```python
from build123d import *

# Parameters (mm, degrees)
SALIENTE_EXTRUIR1_DEPTH = 4
CROQUIS3_W              = 28.5
CROQUIS3_H              = 75
CORTAR_EXTRUIR1_DEPTH   = 135.40982107
CROQUIS4_R              = 2.25
CROQUIS4_R_2            = 2.1
CORTAR_EXTRUIR2_DEPTH   = 135.40982107
CROQUIS5_R              = 25
CORTAR_EXTRUIR3_DEPTH   = 135.40982107
REDONDEO1_R             = 5
CROQUIS6_R              = 2.1
CORTAR_EXTRUIR4_DEPTH   = 135.40982107
CROQUIS7_R              = 2.1
CORTAR_EXTRUIR5_DEPTH   = 135.40982107
CORTAR_EXTRUIR6_REACH   = 136.41
CROQUIS8_R              = 2.1
CROQUIS9_R              = 2.1
CORTAR_EXTRUIR7_DEPTH   = 135.40982107


with BuildPart() as part:
    # Croquis2 → Saliente-Extruir1 (new body)
    with BuildSketch(Plane(origin=(0, 0, 0), x_dir=(1, 0, 0), z_dir=(0, 1, 0))):
        Polygon((-65, 95), (-95, 80), (-95, -95), (95, -95), (95, 80), (65, 95), align=None)
    extrude(amount=SALIENTE_EXTRUIR1_DEPTH)

    # Croquis3 → Cortar-Extruir1 (cut, through all)
    with BuildSketch(Plane(origin=(0, 4, 0), x_dir=(1, 0, 0), z_dir=(0, 1, 0))):
        with Locations((-80.75, 35)):
            Rectangle(CROQUIS3_W, CROQUIS3_H)
        with Locations((80.75, 35)):
            Rectangle(CROQUIS3_W, CROQUIS3_H)
    extrude(amount=-CORTAR_EXTRUIR1_DEPTH, mode=Mode.SUBTRACT)

    # Croquis4 → Cortar-Extruir2 (cut, through all)
    with BuildSketch(Plane(origin=(0, 4, 0), x_dir=(1, 0, 0), z_dir=(0, 1, 0))):
        with Locations(Location((-80.75, -19.5, 0), (0, 0, 270))):
            Circle(CROQUIS4_R)
        with Locations(Location((-80.75, -34.5, 0), (0, 0, 270))):
            Circle(CROQUIS4_R)
        with Locations(Location((-80.75, -49.5, 0), (0, 0, 270))):
            Circle(CROQUIS4_R)
        with Locations(Location((-56.5, 80.75, 0), (0, 0, 270))):
            Circle(CROQUIS4_R_2)
        with Locations(Location((-41.5, 80.75, 0), (0, 0, 270))):
            Circle(CROQUIS4_R_2)
        with Locations(Location((-26.5, 80.75, 0), (0, 0, 270))):
            Circle(CROQUIS4_R_2)
        with Locations(Location((80.75, -49.5, 0), (0, 0, 90))):
            Circle(CROQUIS4_R)
        with Locations(Location((80.75, -34.5, 0), (0, 0, 90))):
            Circle(CROQUIS4_R)
        with Locations(Location((80.75, -19.5, 0), (0, 0, 90))):
            Circle(CROQUIS4_R)
        with Locations(Location((26.5, 80.75, 0), (0, 0, 90))):
            Circle(CROQUIS4_R_2)
        with Locations(Location((41.5, 80.75, 0), (0, 0, 90))):
            Circle(CROQUIS4_R_2)
        with Locations(Location((56.5, 80.75, 0), (0, 0, 90))):
            Circle(CROQUIS4_R_2)
    extrude(amount=-CORTAR_EXTRUIR2_DEPTH, mode=Mode.SUBTRACT)

    # Croquis5 → Cortar-Extruir3 (cut, through all)
    with BuildSketch(Plane(origin=(0, 4, 0), x_dir=(1, 0, 0), z_dir=(0, 1, 0))):
        with Locations(Location((0, 35, 0), (0, 0, 270))):
            Circle(CROQUIS5_R)
        with BuildLine():
            Line((-20, -21.536154127), (-20, -66.536154127))
            ThreePointArc((-20, -66.536154127), (-30, -76.536154127), (-40, -66.536154127))
            Line((-40, -66.536154127), (-40, -21.536154127))
            ThreePointArc((-40, -21.536154127), (-30, -11.536154127), (-20, -21.536154127))
        make_face()
        with BuildLine():
            Line((20, -21.536154127), (20, -66.536154127))
            ThreePointArc((20, -66.536154127), (30, -76.536154127), (40, -66.536154127))
            Line((40, -66.536154127), (40, -21.536154127))
            ThreePointArc((40, -21.536154127), (30, -11.536154127), (20, -21.536154127))
        make_face()
    extrude(amount=-CORTAR_EXTRUIR3_DEPTH, mode=Mode.SUBTRACT)

    # Redondeo1
    # the kernel refuses this fillet: 5 mm, written as the material it adds along each edge
    with BuildSketch(Plane(origin=(-66.5, 4, -72.5), x_dir=(-1, 0, 0), z_dir=(0, -1, 0)), Plane(origin=(-66.5, 4, 2.5), x_dir=(0, 0, -1), z_dir=(0, -1, 0))) as redondeo1_piece_1:
        with BuildLine():
            CenterArc((REDONDEO1_R, -REDONDEO1_R), REDONDEO1_R, 90, 90)
            Line((0, -REDONDEO1_R), (0, 0))
            Line((0, 0), (REDONDEO1_R, 0))
        make_face()
    extrude(amount=4)
    with BuildSketch(Plane(origin=(66.5, 4, -72.5), x_dir=(1, 0, 0), z_dir=(0, -1, 0)), Plane(origin=(66.5, 4, 2.5), x_dir=(0, 0, -1), z_dir=(0, -1, 0))) as redondeo1_piece_2:
        with BuildLine():
            CenterArc((REDONDEO1_R, REDONDEO1_R), REDONDEO1_R, 180, 90)
            Line((0, REDONDEO1_R), (0, 0))
            Line((0, 0), (REDONDEO1_R, 0))
        make_face()
    extrude(amount=4)
    # the kernel refuses this fillet: 5 mm, written as the material it takes off along each edge
    with BuildSketch(Plane(origin=(95, -12.5, 95), x_dir=(0, 0, -1), z_dir=(0, 1, 0)), Plane(origin=(-95, -12.5, 95), x_dir=(1, 0, 0), z_dir=(0, 1, 0)), Plane(origin=(-95, 16.5, -72.5), x_dir=(0, 0, -1), z_dir=(0, -1, 0))) as redondeo1_2_piece_1:
        with BuildLine():
            CenterArc((REDONDEO1_R, REDONDEO1_R), REDONDEO1_R, 180, 90)
            Line((0, REDONDEO1_R), (0, 0))
            Line((0, 0), (REDONDEO1_R, 0))
        make_face()
    extrude(amount=29, mode=Mode.SUBTRACT)
    with BuildSketch(Plane(origin=(-95, -7.725424859, -80), x_dir=(0.894427190999916, 0, -0.447213595499958), z_dir=(0, 1, 0))) as redondeo1_2_piece_2:
        with BuildLine():
            CenterArc((REDONDEO1_R * 0.61803398875, -REDONDEO1_R), REDONDEO1_R, 90, 63.434948823)
            Line((-REDONDEO1_R * 0.27639320225, -REDONDEO1_R * 0.5527864045), (0, 0))
            Line((0, 0), (REDONDEO1_R * 0.61803398875, 0))
        make_face()
    extrude(amount=19.450849719, mode=Mode.SUBTRACT)
    with BuildSketch(Plane(origin=(-65, -2.950849719, -95), x_dir=(1, 0, 0), z_dir=(0, 1, 0)), Plane(origin=(65, -2.950849719, -95), x_dir=(0.8944271909999183, 0, 0.44721359549995315), z_dir=(0, 1, 0))) as redondeo1_2_piece_3:
        with BuildLine():
            CenterArc((REDONDEO1_R * 0.2360679775, -REDONDEO1_R), REDONDEO1_R, 90, 26.565051177)
            Line((-REDONDEO1_R * 0.211145618, -REDONDEO1_R * 0.105572809), (0, 0))
            Line((0, 0), (REDONDEO1_R * 0.2360679775, 0))
        make_face()
    extrude(amount=9.901699437, mode=Mode.SUBTRACT)
    with BuildSketch(Plane(origin=(95, -7.725424859, -80), x_dir=(-0.894427190999915, 0, -0.4472135954999598), z_dir=(0, 1, 0))) as redondeo1_2_piece_4:
        with BuildLine():
            CenterArc((REDONDEO1_R * 0.61803398875, REDONDEO1_R), REDONDEO1_R, 206.565051177, 63.434948823)
            Line((-REDONDEO1_R * 0.27639320225, REDONDEO1_R * 0.5527864045), (0, 0))
            Line((0, 0), (REDONDEO1_R * 0.61803398875, 0))
        make_face()
    extrude(amount=19.450849719, mode=Mode.SUBTRACT)
    with BuildSketch(Plane(origin=(-95, 16.5, 2.5), x_dir=(0, 0, 1), z_dir=(0, -1, 0)), Plane(origin=(95, 16.5, -72.5), x_dir=(0, 0, -1), z_dir=(0, -1, 0)), Plane(origin=(95, 16.5, 2.5), x_dir=(-1, 0, 0), z_dir=(0, -1, 0))) as redondeo1_2_piece_5:
        with BuildLine():
            CenterArc((REDONDEO1_R, -REDONDEO1_R), REDONDEO1_R, 90, 90)
            Line((0, -REDONDEO1_R), (0, 0))
            Line((0, 0), (REDONDEO1_R, 0))
        make_face()
    extrude(amount=29, mode=Mode.SUBTRACT)

    # Croquis6 → Cortar-Extruir4 (cut, through all)
    with BuildSketch(Plane(origin=(0, 4, 0), x_dir=(1, 0, 0), z_dir=(0, 1, 0))):
        with Locations(Location((-57.5, -85, 0), (0, 0, 270))):
            Circle(CROQUIS6_R)
        with Locations(Location((-42.5, -85, 0), (0, 0, 270))):
            Circle(CROQUIS6_R)
        with Locations(Location((42.5, -85, 0), (0, 0, 90))):
            Circle(CROQUIS6_R)
        with Locations(Location((57.5, -85, 0), (0, 0, 90))):
            Circle(CROQUIS6_R)
        with Locations(Location((-7.5, -85, 0), (0, 0, 270))):
            Circle(CROQUIS6_R)
        with Locations(Location((7.5, -85, 0), (0, 0, 270))):
            Circle(CROQUIS6_R)
    extrude(amount=-CORTAR_EXTRUIR4_DEPTH, mode=Mode.SUBTRACT)

    # Croquis7 → Cortar-Extruir5 (cut, through all)
    with BuildSketch(Plane(origin=(0, 4, 0), x_dir=(1, 0, 0), z_dir=(0, 1, 0))):
        with Locations(Location((-57.5, -70, 0), (0, 0, 270))):
            Circle(CROQUIS7_R)
        with Locations(Location((-57.5, -55, 0), (0, 0, 270))):
            Circle(CROQUIS7_R)
        with Locations(Location((57.5, -55, 0), (0, 0, 90))):
            Circle(CROQUIS7_R)
        with Locations(Location((57.5, -70, 0), (0, 0, 90))):
            Circle(CROQUIS7_R)
        with Locations(Location((0, -70, 0), (0, 0, 270))):
            Circle(CROQUIS7_R)
        with Locations(Location((0, -55, 0), (0, 0, 270))):
            Circle(CROQUIS7_R)
    extrude(amount=-CORTAR_EXTRUIR5_DEPTH, mode=Mode.SUBTRACT)

    # Croquis8 → Cortar-Extruir6 (cut, up to next)
    with BuildSketch(Plane.XZ, mode=Mode.PRIVATE) as cortar_extruir6_sk1:
        with Locations(Location((56.5, -57.25, 0), (0, 0, 270))):
            Circle(CROQUIS8_R)
    cortar_extruir6_tool1 = extrude(cortar_extruir6_sk1.sketch, amount=-CORTAR_EXTRUIR6_REACH, mode=Mode.PRIVATE) & part.part
    # Croquis8 → Cortar-Extruir6 (cut, up to next)
    with BuildSketch(Plane.XZ, mode=Mode.PRIVATE) as cortar_extruir6_sk2:
        with Locations(Location((36.5, -57.25, 0), (0, 0, 270))):
            Circle(CROQUIS8_R)
    cortar_extruir6_tool2 = extrude(cortar_extruir6_sk2.sketch, amount=-CORTAR_EXTRUIR6_REACH, mode=Mode.PRIVATE) & part.part
    # Croquis8 → Cortar-Extruir6 (cut, up to next)
    with BuildSketch(Plane.XZ, mode=Mode.PRIVATE) as cortar_extruir6_sk3:
        with Locations(Location((56.5, -12.75, 0), (0, 0, 90))):
            Circle(CROQUIS8_R)
    cortar_extruir6_tool3 = extrude(cortar_extruir6_sk3.sketch, amount=-CORTAR_EXTRUIR6_REACH, mode=Mode.PRIVATE) & part.part
    # Croquis8 → Cortar-Extruir6 (cut, up to next)
    with BuildSketch(Plane.XZ, mode=Mode.PRIVATE) as cortar_extruir6_sk4:
        with Locations(Location((36.5, -12.75, 0), (0, 0, 90))):
            Circle(CROQUIS8_R)
    cortar_extruir6_tool4 = extrude(cortar_extruir6_sk4.sketch, amount=-CORTAR_EXTRUIR6_REACH, mode=Mode.PRIVATE) & part.part
    # Croquis8 → Cortar-Extruir6 (cut, up to next)
    with BuildSketch(Plane.XZ, mode=Mode.PRIVATE) as cortar_extruir6_sk5:
        with Locations(Location((-36.5, -12.75, 0), (0, 0, 270))):
            Circle(CROQUIS8_R)
    cortar_extruir6_tool5 = extrude(cortar_extruir6_sk5.sketch, amount=-CORTAR_EXTRUIR6_REACH, mode=Mode.PRIVATE) & part.part
    # Croquis8 → Cortar-Extruir6 (cut, up to next)
    with BuildSketch(Plane.XZ, mode=Mode.PRIVATE) as cortar_extruir6_sk6:
        with Locations(Location((-56.5, -12.75, 0), (0, 0, 270))):
            Circle(CROQUIS8_R)
    cortar_extruir6_tool6 = extrude(cortar_extruir6_sk6.sketch, amount=-CORTAR_EXTRUIR6_REACH, mode=Mode.PRIVATE) & part.part
    # Croquis8 → Cortar-Extruir6 (cut, up to next)
    with BuildSketch(Plane.XZ, mode=Mode.PRIVATE) as cortar_extruir6_sk7:
        with Locations(Location((-36.5, -57.25, 0), (0, 0, 90))):
            Circle(CROQUIS8_R)
    cortar_extruir6_tool7 = extrude(cortar_extruir6_sk7.sketch, amount=-CORTAR_EXTRUIR6_REACH, mode=Mode.PRIVATE) & part.part
    # Croquis8 → Cortar-Extruir6 (cut, up to next)
    with BuildSketch(Plane.XZ, mode=Mode.PRIVATE) as cortar_extruir6_sk8:
        with Locations(Location((-56.5, -57.25, 0), (0, 0, 90))):
            Circle(CROQUIS8_R)
    cortar_extruir6_tool8 = extrude(cortar_extruir6_sk8.sketch, amount=-CORTAR_EXTRUIR6_REACH, mode=Mode.PRIVATE) & part.part
    add(cortar_extruir6_tool1.solids().sort_by_distance((56.5, 0, -57.25))[0], mode=Mode.SUBTRACT)
    add(cortar_extruir6_tool2.solids().sort_by_distance((36.5, 0, -57.25))[0], mode=Mode.SUBTRACT)
    add(cortar_extruir6_tool3.solids().sort_by_distance((56.5, 0, -12.75))[0], mode=Mode.SUBTRACT)
    add(cortar_extruir6_tool4.solids().sort_by_distance((36.5, 0, -12.75))[0], mode=Mode.SUBTRACT)
    add(cortar_extruir6_tool5.solids().sort_by_distance((-36.5, 0, -12.75))[0], mode=Mode.SUBTRACT)
    add(cortar_extruir6_tool6.solids().sort_by_distance((-56.5, 0, -12.75))[0], mode=Mode.SUBTRACT)
    add(cortar_extruir6_tool7.solids().sort_by_distance((-36.5, 0, -57.25))[0], mode=Mode.SUBTRACT)
    add(cortar_extruir6_tool8.solids().sort_by_distance((-56.5, 0, -57.25))[0], mode=Mode.SUBTRACT)

    # Croquis9 → Cortar-Extruir7 (cut, through all)
    with BuildSketch(Plane(origin=(0, 4, 0), x_dir=(1, 0, 0), z_dir=(0, 1, 0))):
        with Locations(Location((-7.5, 80.75, 0), (0, 0, 270))):
            Circle(CROQUIS9_R)
        with Locations(Location((7.5, 80.75, 0), (0, 0, 270))):
            Circle(CROQUIS9_R)
    extrude(amount=-CORTAR_EXTRUIR7_DEPTH, mode=Mode.SUBTRACT)


solid = part.part
```
The listing builds one solid part. Answer for the finished solid, in the listing's coordinates (mm). A direction names the side the tool comes from. Coordinates: 2 decimals unless noted, no trailing zeros. Write each loop counter-clockwise with the first axis right and the second up, starting at its lowest first coordinate (ties: lowest second). Pieces come first, ordered by that corner, then holes.
Q1. The mould has two halves that part along X. Classify faces 1 (the cylindrical face through (93.47, 2.03, -73.9)), 2 (the cylindrical face through (-7.41, 2.03, 82.9)), 3 (the cylindrical face through (-68, 2.03, -71.07)): released by +X, released by -X, zero draft, split by the parting line, or undercut.
Returned:
face 1: released by +X
face 2: undercut
face 3: released by -X
Q2. Given P1, Ø3.5, axis at x = 7.5, z = -80.75, coming from the -Y side; P2, Ø1, axis at y = 3, z = -68, coming from the -X side, each flat-ended and moving along its own axis, determine where each tip first touches the part or whether it passes through.
Returned:
P1: passes through
P2: stops at x = -66.6
Q3. Which of the six approach directions +Z, -Z, +X, -X, +Y, -Y give full straight-line access (tool end or side, diameter ignored) to faces 4 (the cylindrical face through (-94, 2, 93)), 5 (the cylindrical face through (-29.78, 2.028, 76.534))?
Returned:
face 4: +Z, -X, +Y, -Y
face 5: +Y, -Y
Q4. Section B-B, the plane z = -19 is taken. Write down the section's boundary in (x, y), then the cut area to 3 significant figures.
Returned:
outline: (-66.5, 0) - (-19.21, 0) - (-19.21, 4) - (-66.5, 4) - close; (19.21, 0) - (66.5, 0) - (66.5, 4) - (19.21, 4) - close
area: 378 mm2
Q5. Find the intervals of material crossed by line 1 along X through (y, z) = (3.5, 30.5); line 2 along Z through (x, y) = (80.75, 2.1) (3 decimals); line 3 along X through (y, z) = (1.45, 19.5), in increasing order.
Returned:
line 1: x = -95 to -40, -20 to 20, 40 to 95
line 2: z = -87.125 to -72.5, 2.5 to 17.25, 21.75 to 32.25, 36.75 to 47.25, 51.75 to 95
line 3: x = -95 to -83, -78.5 to -39.79, -20.21 to 20.21, 39.79 to 78.5, 83 to 95
Q6. Section A-A, the plane z = 24.5 is taken. Write down the section's boundary in (x, y), then the cut area to 3 significant figures.
Returned:
outline: (-95, 0) - (-40, 0) - (-40, 4) - (-95, 4) - close; (-20, 0) - (20, 0) - (20, 4) - (-20, 4) - close; (40, 0) - (95, 0) - (95, 4) - (40, 4) - close
area: 600 mm2
Q7. Section C-C, the plane y = 1.55 is taken. Give the number of separate pieces and of enclosed holes in the cut face, then the cut area to 3 significant figures.
Returned:
separate pieces: 1
enclosed holes: 37
area: 26,500 mm2
Q8. Section D-D, the plane z = -49 is taken. Write down the section's boundary in (x, y).
Returned:
outline: (-66.5, 0) - (-20.71, 0) - (-20.71, 4) - (-66.5, 4) - close; (20.71, 0) - (66.5, 0) - (66.5, 4) - (20.71, 4) - close
